Design review of the part built by this model. Coordinates are the model's own, in mm. Face numbers are marked on the shaded views. A direction names the side the tool comes from. Coordinates: 2 decimals unless noted, no trailing zeros. Write each loop counter-clockwise with the first axis right and the second up, starting at its lowest first coordinate (ties: lowest second). Pieces come first, ordered by that corner, then holes. Notation, with made-up numbers: (17, 23) - (43, 23) arc R36 ccw to (43, 60) - close; hole circle Ø10 at (35, 38.25). An arc over 180 degrees is marked (long way). Answer as a JSON object with one key per item and string values.
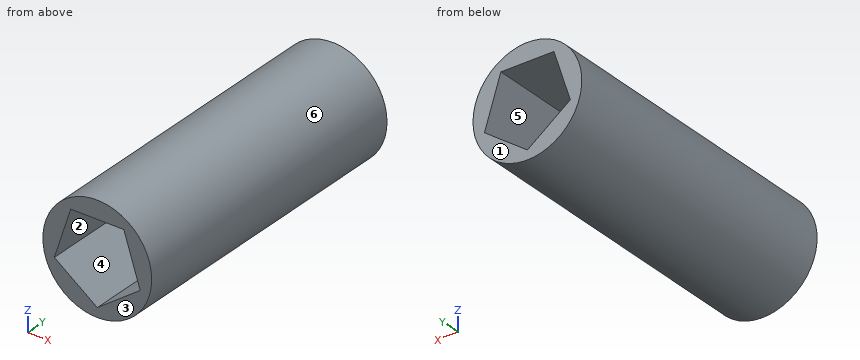
```python
from build123d import *

# Parameters (mm, degrees)
SKETCH1_R           = 3.5
BOSS_EXTRUDE1_DEPTH = 20


with BuildPart() as part:
    # Sketch1 → Boss-Extrude1 (new body)
    with BuildSketch(Plane(origin=(0, 0, 0), x_dir=(1, 0, 0), z_dir=(0, 1, 0))):
        Circle(SKETCH1_R)
        Polygon((1.707374941, -2.35), (2.762590686, 0.897620126), (0, 2.904759747), (-2.762590686, 0.897620126), (-1.707374941, -2.35), align=None, mode=Mode.SUBTRACT)
    extrude(amount=BOSS_EXTRUDE1_DEPTH)


solid = part.part
```
(1) Take a section at A-A, the plane z = -2.25. Write out the cut boundary in (x, y), and give its area (3 significant figures).
Solved:
{"outline": "(-2.68, 0) - (-0.9, 0) - (-0.9, 20) - (-2.68, 20) - close; (0.9, 0) - (2.68, 0) - (2.68, 20) - (0.9, 20) - close", "area": "71.2 mm^2"}
(2) Take a section at C-C, the plane x = -2.5. Write out the cut boundary in (y, z), and give its area (3 significant figures).
Solved:
{"outline": "(0, -2.45) - (20, -2.45) - (20, -1.09) - (0, -1.09) - close; (0, -0.09) - (20, -0.09) - (20, 2.45) - (0, 2.45) - close", "area": "78.0 mm^2"}
(3) Take a section at B-B, the plane y = 7.25. Write out the cut boundary in (x, z), and give its area (3 significant figures).
Solved:
{"outline": "circle Ø7 at (0, 0); hole (-2.76, -0.9) - (0, -2.9) - (2.76, -0.9) - (1.71, 2.35) - (-1.71, 2.35) - close", "area": "18.4 mm^2"}
(4) Tool access review of the marked faces 1 and 2: name each direction out of +Z, -Z, +X, -X, +Y, -Y from which nothing blocks a thin tool from reaching the whole face with its end or side.
Solved:
{"face 1": "+Z, -Z, +X, -X, +Y", "face 2": "+Y, -Y"}
(5) The part is to be moulded in two halves that separate along Z. For the marked faces 3, 4, 5 and 6, say which applies: pulls with the +Z half, pulls with the -Z half, needs draft (parallel to the pull), parting line crosses it, or undercut.
Solved:
{"face 3": "needs draft", "face 4": "undercut", "face 5": "undercut", "face 6": "parting line crosses it"}
(6) Take a section at D-D, the plane x = 3.25. Write out the cut boundary in (y, z).
Solved:
{"outline": "(0, -1.3) - (20, -1.3) - (20, 1.3) - (0, 1.3) - close"}
(7) To check wall thickness, follow line 1 (Z direction, x = -1.5, y = 11.25); line 2 (X direction, y = 12.25, z = -0.75); line 3 (Z direction, x = -0.75, y = 8.5). State the ranges of each line that lie inside material, in increasing order. Write a range as from..to.
Solved:
{"line 1": "z = -3.16..-1.81, 2.35..3.16", "line 2": "x = -3.42..-2.71, 2.71..3.42", "line 3": "z = -3.42..-2.36, 2.35..3.42"}
(8) For pin 1 (4 mm diameter, centred on x = 0.5, z = 2, fed in from -Y); pin 2 (2 mm diameter, centred on y = 5.5, z = 2.5, fed in from +X); pin 3 (1.5 mm diameter, centred on y = 5.5, z = 1.5, fed in from +X); pin 4 (2 mm diameter, centred on x = 2.5, y = 4, fed in from -Z), all flat-tipped, find the tip position at first contact; note any pin that passes through.
Solved:
{"pin 1": "stops at y = 0", "pin 2": "stops at x = 3.16", "pin 3": "stops at x = 3.42", "pin 4": "stops at z = -3.16"}
